```python
from build123d import *

# Parameters (mm, degrees)
F0_R     = 4
F1_DEPTH = 5


with BuildPart() as f1:
    # F0 (on Front) → F1 (new body)
    with BuildSketch(Plane.XZ):
        with BuildLine():
            Line((5.4, 0.3), (5.992495, 0.3))
            ThreePointArc((5.992495, 0.3), (5.884712, 1.170542), (5.651149, 2.016065))
            Line((5.651149, 2.016065), (5.103755, 1.789327))
            ThreePointArc((5.103755, 1.789327), (4.157458, 1.722075), (4.874144, 2.343654))
            Line((4.874144, 2.343654), (5.421539, 2.570393))
            ThreePointArc((5.421539, 2.570393), (4.988818, 3.333421), (4.449466, 4.025202))
            Line((4.449466, 4.025202), (4.030509, 3.606245))
            ThreePointArc((4.030509, 3.606245), (4.034276, 3.570978), (4.035534, 3.535534))
            ThreePointArc((4.035534, 3.535534), (3.157807, 3.207933), (3.606245, 4.030509))
            Line((3.606245, 4.030509), (4.025202, 4.449466))
            ThreePointArc((4.025202, 4.449466), (3.333421, 4.988818), (2.570393, 5.421539))
            Line((2.570393, 5.421539), (2.343654, 4.874144))
            ThreePointArc((2.343654, 4.874144), (2.395661, 4.751461), (2.413417, 4.619398))
            ThreePointArc((2.413417, 4.619398), (1.60686, 4.224401), (1.789327, 5.103755))
            Line((1.789327, 5.103755), (2.016065, 5.651149))
            ThreePointArc((2.016065, 5.651149), (1.170542, 5.884712), (0.3, 5.992495))
            Line((0.3, 5.992495), (0.3, 5.4))
            ThreePointArc((0.3, 5.4), (0.447214, 5.223607), (0.5, 5))
            ThreePointArc((0.5, 5), (-0.223607, 4.552786), (-0.3, 5.4))
            Line((-0.3, 5.4), (-0.3, 5.992495))
            ThreePointArc((-0.3, 5.992495), (-1.170542, 5.884712), (-2.016065, 5.651149))
            Line((-2.016065, 5.651149), (-1.789327, 5.103755))
            ThreePointArc((-1.789327, 5.103755), (-1.51842, 4.925955), (-1.413417, 4.619398))
            ThreePointArc((-1.413417, 4.619398), (-2.04548, 4.137154), (-2.343654, 4.874144))
            Line((-2.343654, 4.874144), (-2.570393, 5.421539))
            ThreePointArc((-2.570393, 5.421539), (-3.333421, 4.988818), (-4.025202, 4.449466))
            Line((-4.025202, 4.449466), (-3.606245, 4.030509))
            ThreePointArc((-3.606245, 4.030509), (-3.207933, 3.913261), (-3.035534, 3.535534))
            ThreePointArc((-3.035534, 3.535534), (-3.570978, 3.036792), (-4.030509, 3.606245))
            Line((-4.030509, 3.606245), (-4.449466, 4.025202))
            ThreePointArc((-4.449466, 4.025202), (-4.988818, 3.333421), (-5.421539, 2.570393))
            Line((-5.421539, 2.570393), (-4.874144, 2.343654))
            ThreePointArc((-4.874144, 2.343654), (-4.371782, 2.347798), (-4.119398, 1.913417))
            ThreePointArc((-4.119398, 1.913417), (-4.556861, 1.417343), (-5.103755, 1.789327))
            Line((-5.103755, 1.789327), (-5.651149, 2.016065))
            ThreePointArc((-5.651149, 2.016065), (-5.884712, 1.170542), (-5.992495, 0.3))
            Line((-5.992495, 0.3), (-5.4, 0.3))
            ThreePointArc((-5.4, 0.3), (-4.841886, 0.474342), (-4.5, 0))
            ThreePointArc((-4.5, 0), (-4.841886, -0.474342), (-5.4, -0.3))
            Line((-5.4, -0.3), (-5.992495, -0.3))
            ThreePointArc((-5.992495, -0.3), (-5.884712, -1.170542), (-5.651149, -2.016065))
            Line((-5.651149, -2.016065), (-5.103755, -1.789327))
            ThreePointArc((-5.103755, -1.789327), (-4.556861, -1.417343), (-4.119398, -1.913417))
            ThreePointArc((-4.119398, -1.913417), (-4.371782, -2.347798), (-4.874144, -2.343654))
            Line((-4.874144, -2.343654), (-5.421539, -2.570393))
            ThreePointArc((-5.421539, -2.570393), (-4.988818, -3.333421), (-4.449466, -4.025202))
            Line((-4.449466, -4.025202), (-4.030509, -3.606245))
            ThreePointArc((-4.030509, -3.606245), (-3.570978, -3.036792), (-3.035534, -3.535534))
            ThreePointArc((-3.035534, -3.535534), (-3.207933, -3.913261), (-3.606245, -4.030509))
            Line((-3.606245, -4.030509), (-4.025202, -4.449466))
            ThreePointArc((-4.025202, -4.449466), (-3.333421, -4.988818), (-2.570393, -5.421539))
            Line((-2.570393, -5.421539), (-2.343654, -4.874144))
            ThreePointArc((-2.343654, -4.874144), (-2.04548, -4.137154), (-1.413417, -4.619398))
            ThreePointArc((-1.413417, -4.619398), (-1.51842, -4.925955), (-1.789327, -5.103755))
            Line((-1.789327, -5.103755), (-2.016065, -5.651149))
            ThreePointArc((-2.016065, -5.651149), (-1.170542, -5.884712), (-0.3, -5.992495))
            Line((-0.3, -5.992495), (-0.3, -5.4))
            ThreePointArc((-0.3, -5.4), (-0.223607, -4.552786), (0.5, -5))
            ThreePointArc((0.5, -5), (0.447214, -5.223607), (0.3, -5.4))
            Line((0.3, -5.4), (0.3, -5.992495))
            ThreePointArc((0.3, -5.992495), (1.170542, -5.884712), (2.016065, -5.651149))
            Line((2.016065, -5.651149), (1.789327, -5.103755))
            ThreePointArc((1.789327, -5.103755), (1.60686, -4.224401), (2.413417, -4.619398))
            ThreePointArc((2.413417, -4.619398), (2.395661, -4.751461), (2.343654, -4.874144))
            Line((2.343654, -4.874144), (2.570393, -5.421539))
            ThreePointArc((2.570393, -5.421539), (3.333421, -4.988818), (4.025202, -4.449466))
            Line((4.025202, -4.449466), (3.606245, -4.030509))
            ThreePointArc((3.606245, -4.030509), (3.157807, -3.207933), (4.035534, -3.535534))
            ThreePointArc((4.035534, -3.535534), (4.034276, -3.570978), (4.030509, -3.606245))
            Line((4.030509, -3.606245), (4.449466, -4.025202))
            ThreePointArc((4.449466, -4.025202), (4.988818, -3.333421), (5.421539, -2.570393))
            Line((5.421539, -2.570393), (4.874144, -2.343654))
            ThreePointArc((4.874144, -2.343654), (4.157458, -1.722075), (5.103755, -1.789327))
            Line((5.103755, -1.789327), (5.651149, -2.016065))
            ThreePointArc((5.651149, -2.016065), (5.884712, -1.170542), (5.992495, -0.3))
            Line((5.992495, -0.3), (5.4, -0.3))
            ThreePointArc((5.4, -0.3), (4.5, 0), (5.4, 0.3))
        make_face()
        Circle(F0_R, mode=Mode.SUBTRACT)
    extrude(amount=F1_DEPTH)


solid = f1.part
```
Build history of the part. All positions in model axes, mm. Coordinates: 2 decimals unless noted, no trailing zeros. Order: outer loops, then holes, each group sorted by start corner. A loop starts at its lowest first (then second) coordinate and runs counter-clockwise, first axis right, second up. Notation, with made-up numbers: (-4.5, 5.5) -> (36.5, 5.5) arc R18 cw to (36.5, 11.5) -> close; hole circle Ø1 at (22.25, 8). An arc over 180 degrees is marked (long way). Answer in a Markdown table with one row per item. Add a question column.
Q1. Band-saw the part on D-D, the plane x = -1.25. List the corners of the cut face in (y, z), then the cut area to 3 significant figures.
Q2. Wall check: line 1 along Z through (x, y) = (0, -0.95); line 2 along X through (y, z) = (-3.9, -5); line 3 along Z through (x, y) = (5.25, -1.25). Give the ranges that are in metal, low to high. Write a range as [from, to].
Q3. Band-saw the part on C-C, the plane x = 3.75. List the corners of the cut face in (y, z), then the cut area to 3 significant figures.
Q4. Band-saw the part on A-A, the plane x = 0. List the corners of the cut face in (y, z), then the cut area to 3 significant figures.
Q5. Drop flat-ended pins along their axis: pin 1 (2 mm diameter, centred on x = -2.5, z = -1.5, fed in from -Y) (1 decimal); pin 2 (1 mm diameter, centred on x = 1.5, y = -1, fed in from +Z); pin 3 (0.5 mm diameter, centred on x = -5.5, y = -2.5, fed in from +Z). Give the stop position or say it passes through.
Q6. Mould opens along Z. For faces 1 (the face through (4.5, -2.5, 0)), 2 (the face through (4.982, -2.465, -3.344)), 3 (the face through (3.344, -2.465, 4.982)), 4 (the face through (-1.42, -5, -3.91)) say: +Z half, -Z half, draft (parallel to the pull), parting line (faces both ways), or undercut.
Q7. Band-saw the part on B-B, the plane z = 3.25. List the corners of the cut face in (x, y), then the cut area to 3 significant figures.
Answers follow:
| question | item | result |
|---|---|---|
| 1 | outline | (-5, -5.87) -> (0, -5.87) -> (0, -3.8) -> (-5, -3.8) -> close; (-5, 3.8) -> (0, 3.8) -> (0, 5.87) -> (-5, 5.87) -> close |
| 1 | area | 20.7 mm^2 |
| 2 | line 1 | [-4.5, -4], [4, 4.5] |
| 2 | line 2 | [-3.32, -2.4], [-1.59, -0.5], [0.5, 1.59], [2.4, 3.32] |
| 2 | line 3 | [-2.9, -2.5], [-1.85, -0.43], [0.43, 1.85], [2.5, 2.9] |
| 3 | outline | (-5, -4.68) -> (0, -4.68) -> (0, -4.17) -> (-5, -4.17) -> close; (-5, -3.08) -> (0, -3.08) -> (0, -1.39) -> (-5, -1.39) -> close; (-5, 1.39) -> (0, 1.39) -> (0, 3.08) -> (-5, 3.08) -> close; (-5, 4.17) -> (0, 4.17) -> (0, 4.68) -> (-5, 4.68) -> close |
| 3 | area | 22.0 mm^2 |
| 4 | outline | (-5, -4.5) -> (0, -4.5) -> (0, -4) -> (-5, -4) -> close; (-5, 4) -> (0, 4) -> (0, 4.5) -> (-5, 4.5) -> close |
| 4 | area | 5.00 mm^2 |
| 5 | pin 1 | through |
| 5 | pin 2 | z = 5.92 |
| 5 | pin 3 | z = 2.9 |
| 6 | face 1 | undercut |
| 6 | face 2 | -Z half |
| 6 | face 3 | +Z half |
| 6 | face 4 | draft |
| 7 | outline | (-5.04, -5) -> (-3.95, -5) -> (-3.95, 0) -> (-5.04, 0) -> close; (-3.13, -5) -> (-2.33, -5) -> (-2.33, 0) -> (-3.13, 0) -> close; (2.33, -5) -> (3.13, -5) -> (3.13, 0) -> (2.33, 0) -> close; (3.95, -5) -> (5.04, -5) -> (5.04, 0) -> (3.95, 0) -> close |
| 7 | area | 18.9 mm^2 |
